Verification items for the finished model (mm, model axes). Face numbers are marked on the shaded views. A direction names the side the tool comes from. Coordinates: 2 decimals unless noted, no trailing zeros. Loops run counter-clockwise (first coordinate to the right, second up) from the corner with the lowest first, then second, coordinate; pieces in that order, holes last. Notation, with made-up numbers: (15, -23.5) -> (45, -23.5) arc R19 ccw to (45, 3.5) -> close; hole circle Ø5 at (63.5, 11). An arc over 180 degrees is marked (long way). Answer as a JSON object with one key per item and string values. Group by question number.
Q1. Set-up check for the marked faces 5, 6 and 7: record each of +Z, -Z, +X, -X, +Y, -Y from which the full face is reachable in a straight line by a thin tool's end or side.
Q2. Release check for a two-part mould opening along Y. For the marked faces 1, 2, 3 and 4 record: released by +Y, released by -Y, zero draft, split by the parting line, or undercut.
Q3. Cross-section at C-C on z = -4.25. Record the boundary of the cut face in (x, y).
Q4. Cross-section at A-A on x = -14. Record the boundary of the cut face in (y, z) (3 decimals).
Q5. Cross-section at D-D on x = -0.95. Record the boundary of the cut face in (y, z).
Q6. Scan lines: L1, parallel to Z at x = -14, y = 16.95 (3 decimals); L2, parallel to Y at x = -1, z = -5; L3, parallel to X at y = 17, z = 0 (3 decimals). Record each from-to range of solid material in increasing order.
Q7. Gauge pin test, flat ends, axial feed: pin 1 Ø1.5 at (x, z) = (12.5, 0) entering from -Y; pin 2 Ø1.2 at (x, y) = (12, 4.5) entering from +Z; pin 3 Ø0.5 at (x, y) = (12.5, 4.5) entering from -Z. Record the tip position at first contact, or that the pin passes through.
Q8. Cross-section at B-B on y = 4.5. Record the boundary of the cut face in (x, z).
```python
from build123d import *

# Parameters (mm, degrees)
ESBO_O1_W                = 22.6
ESBO_O1_H                = 12.3
RESSALTO_EXTRUS_O1_DEPTH = 22.4
ESBO_O2_W                = 12.3
ESBO_O2_H                = 2.3
RESSALTO_EXTRUS_O2_DEPTH = 4.8
CORTE_EXTRUS_O1_DEPTH    = 26.13806874
RESSALTO_EXTRUS_O3_DEPTH = 4.2
ESBO_O5_R                = 2.4
RESSALTO_EXTRUS_O4_DEPTH = 3.2
ESBO_O6_W                = 3.7
ESBO_O6_H                = 1.1
RESSALTO_EXTRUS_O5_DEPTH = 3


with BuildPart() as part:
    # Esboço1 → Ressalto-extrusão1 (new body)
    with BuildSketch(Plane(origin=(0, 0, 0), x_dir=(1, 0, 0), z_dir=(0, 1, 0))):
        Rectangle(ESBO_O1_W, ESBO_O1_H)
    extrude(amount=RESSALTO_EXTRUS_O1_DEPTH)

    # Esboço2 → Ressalto-extrusão2 (add)
    with BuildSketch(Plane(origin=(11.3, 0, 0), x_dir=(0, 0, -1), z_dir=(1, 0, 0))):
        with Locations((0, 17.15)):
            Rectangle(ESBO_O2_W, ESBO_O2_H)
    ressalto_extrus_o2 = extrude(amount=RESSALTO_EXTRUS_O2_DEPTH)

    # Esboço3 → Corte-extrusão1 (cut, through all)
    with BuildSketch(Plane(origin=(0, 18.3, 0), x_dir=(1, 0, 0), z_dir=(0, 1, 0))):
        with BuildLine():
            Line((14.856227189, 0.65), (16.1, 0.65))
            Line((16.1, 0.65), (16.1, -0.65))
            Line((16.1, -0.65), (14.856227189, -0.65))
            ThreePointArc((14.856227189, -0.65), (12.925, 0), (14.856227189, 0.65))
        make_face()
    corte_extrus_o1 = extrude(amount=-CORTE_EXTRUS_O1_DEPTH, mode=Mode.SUBTRACT)

    # Espelhar1: Ressalto-extrusão2, Corte-extrusão1 across plane
    add(ressalto_extrus_o2.mirror(Plane(origin=(0, 0, 0), x_dir=(0, 0, 1), z_dir=(1, 0, 0))))
    add(corte_extrus_o1.mirror(Plane(origin=(0, 0, 0), x_dir=(0, 0, 1), z_dir=(1, 0, 0))), mode=Mode.SUBTRACT)

    # Esboço4 → Ressalto-extrusão3 (add)
    with BuildSketch(Plane(origin=(0, 22.4, 0), x_dir=(1, 0, 0), z_dir=(0, 1, 0))):
        with BuildLine():
            ThreePointArc((-0.424590164, -2.597391866), (11.3, 0), (-0.424590164, 2.597391866))
            ThreePointArc((-0.424590164, 2.597391866), (-3.6, 0), (-0.424590164, -2.597391866))
        make_face()
    extrude(amount=RESSALTO_EXTRUS_O3_DEPTH)

    # Esboço5 → Ressalto-extrusão4 (add)
    with BuildSketch(Plane(origin=(0, 26.6, 0), x_dir=(1, 0, 0), z_dir=(0, 1, 0))):
        with Locations(Location((5.15, 0, 0), (0, 0, 270))):
            Circle(ESBO_O5_R)
    extrude(amount=RESSALTO_EXTRUS_O4_DEPTH)

    # Esboço6 → Ressalto-extrusão5 (add)
    with BuildSketch(Plane(origin=(11.3, 0, 0), x_dir=(0, 0, -1), z_dir=(1, 0, 0))):
        with Locations((0, 4.55)):
            Rectangle(ESBO_O6_W, ESBO_O6_H)
    extrude(amount=RESSALTO_EXTRUS_O5_DEPTH)


solid = part.part
```
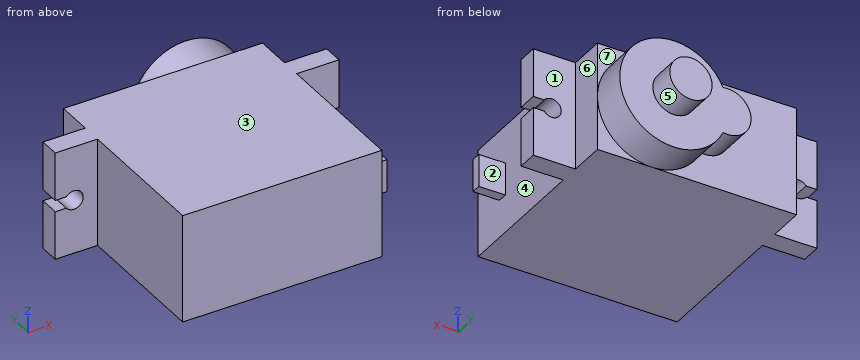
Computed values:
{
 "1": {"face 5": "+Y", "face 6": "+Z, -Z, +X, +Y", "face 7": "+Z, +X, +Y"},
 "2": {"face 1": "released by +Y", "face 2": "undercut", "face 3": "zero draft", "face 4": "undercut"},
 "3": {"outline": "(-16.1, 16) -> (-11.3, 16) -> (-11.3, 0) -> (11.3, 0) -> (11.3, 16) -> (16.1, 16) -> (16.1, 18.3) -> (11.3, 18.3) -> (11.3, 22.4) -> (9.6, 22.4) -> (9.6, 26.6) -> (0.7, 26.6) -> (0.7, 22.4) -> (-11.3, 22.4) -> (-11.3, 18.3) -> (-16.1, 18.3) -> close"},
 "4": {"outline": "(16, -6.15) -> (18.3, -6.15) -> (18.3, -1.075) -> (16, -1.075) -> close; (16, 1.075) -> (18.3, 1.075) -> (18.3, 6.15) -> (16, 6.15) -> close"},
 "5": {"outline": "(0, -6.15) -> (22.4, -6.15) -> (22.4, -2.65) -> (26.6, -2.65) -> (26.6, 2.65) -> (22.4, 2.65) -> (22.4, 6.15) -> (0, 6.15) -> close"},
 "6": {"L1": "z = -6.15 to -1.075, 1.075 to 6.15", "L2": "y = 0 to 22.4", "L3": "x = -12.925 to 12.925"},
 "7": {"pin 1": "stops at y = 4", "pin 2": "stops at z = 1.85", "pin 3": "stops at z = -1.85"},
 "8": {"outline": "(-11.3, -6.15) -> (11.3, -6.15) -> (11.3, -1.85) -> (14.3, -1.85) -> (14.3, 1.85) -> (11.3, 1.85) -> (11.3, 6.15) -> (-11.3, 6.15) -> close"}
}
